```python
from build123d import *

# Parameters (mm, degrees)
BOSS_EXTRUDE1_DEPTH = 30
BOSS_EXTRUDE3_DEPTH = 5
BOSS_EXTRUDE4_DEPTH = 60
BOSS_EXTRUDE5_DEPTH = 5
RIB2_REACH          = 93.092
SKETCH12_WALL_W     = 244.715003534
SKETCH12_WALL_H     = 1.5
RIB4_REACH          = 88.249
SKETCH15_WALL_W     = 235.02855303
SKETCH15_WALL_H     = 1.5
FILLET2_R           = 6
FILLET3_R           = 3
FILLET4_R           = 5
FILLET6_R           = 1
CUT_EXTRUDE4_DEPTH  = 88.321245983
SKETCH17_R          = 12.5
CUT_EXTRUDE5_DEPTH  = 5
FILLET7_R           = 1
FILLET8_R           = 1


with BuildPart() as part:
    # Sketch1 → Boss-Extrude1 (new body)
    with BuildSketch(Plane.XY):
        Polygon((0, 0), (0, 50), (-12.5, 50), (-12.5, 25.213498553), (-10.5, 25.213498553), (-10.5, 48), (-6.7, 48), (-4, 43.5), (-4, 0), align=None)
    extrude(amount=BOSS_EXTRUDE1_DEPTH)

    # Sketch2 → Boss-Extrude3 (add)
    with BuildSketch(Plane(origin=(0, 0, 0), x_dir=(0, 0, -1), z_dir=(1, 0, 0))):
        with BuildLine():
            Line((-30, 20), (-30, 29.013878189))
            ThreePointArc((-30, 29.013878189), (-15, 37.5), (0, 29.013878189))
            Line((0, 29.013878189), (0, 20))
            Line((0, 20), (0, 10.986121811))
            ThreePointArc((0, 10.986121811), (-15, 2.5), (-30, 10.986121811))
            Line((-30, 10.986121811), (-30, 20))
        make_face()
    extrude(amount=BOSS_EXTRUDE3_DEPTH)

    # Sketch8 → Boss-Extrude4 (add)
    with BuildSketch(Plane(origin=(5, 0, 0), x_dir=(0, 0, -1), z_dir=(1, 0, 0))):
        with BuildLine():
            Line((-15.593853911, 21.273523821), (-14.406146089, 21.273523821))
            Line((-14.406146089, 21.273523821), (-8.660726074, 33.594616806))
            ThreePointArc((-8.660726074, 33.594616806), (-1.141807012, 25.740251485), (-0.904610688, 14.86969785))
            Line((-0.904610688, 14.86969785), (-10.032290508, 18.191901612))
            Line((-10.032290508, 18.191901612), (-19.967709492, 18.191901612))
            Line((-19.967709492, 18.191901612), (-29.095389312, 14.86969785))
            ThreePointArc((-29.095389312, 14.86969785), (-28.858192988, 25.740251485), (-21.339273926, 33.594616806))
            Line((-21.339273926, 33.594616806), (-15.593853911, 21.273523821))
        make_face()
    extrude(amount=BOSS_EXTRUDE4_DEPTH)

    # Sketch9 → Boss-Extrude5 (add)
    with BuildSketch(Plane(origin=(65, 0, 0), x_dir=(0, 0, -1), z_dir=(1, 0, 0))):
        with BuildLine():
            Line((-21.339273926, 33.594616806), (-22.39581958, 35.860386273))
            ThreePointArc((-22.39581958, 35.860386273), (-26.709477013, 33.005312303), (-30, 29.013878189))
            Line((-30, 29.013878189), (-27.857142857, 27.726181305))
            ThreePointArc((-27.857142857, 27.726181305), (-29.930908857, 21.438040583), (-29.095389312, 14.86969785))
            Line((-29.095389312, 14.86969785), (-19.967709492, 18.191901612))
            Line((-19.967709492, 18.191901612), (-10.032290508, 18.191901612))
            Line((-10.032290508, 18.191901612), (-0.904610688, 14.86969785))
            ThreePointArc((-0.904610688, 14.86969785), (-0.069091143, 21.438040583), (-2.142857143, 27.726181305))
            Line((-2.142857143, 27.726181305), (0, 29.013878189))
            ThreePointArc((0, 29.013878189), (-3.290522987, 33.005312303), (-7.60418042, 35.860386273))
            Line((-7.60418042, 35.860386273), (-8.660726074, 33.594616806))
            Line((-8.660726074, 33.594616806), (-14.406146089, 21.273523821))
            Line((-14.406146089, 21.273523821), (-15.593853911, 21.273523821))
            Line((-15.593853911, 21.273523821), (-21.339273926, 33.594616806))
        make_face()
    extrude(amount=BOSS_EXTRUDE5_DEPTH)

    # Sketch12 wall → Rib2 (add, up to next)
    with BuildSketch(Plane(origin=(35, 12.772029248, 23.163468829), x_dir=(0.991227900683, 0.1241932725, 0.045202654495), z_dir=(-0.132163720089, 0.931449543789, 0.33901990866)), mode=Mode.PRIVATE) as rib2_sk1:
        Rectangle(SKETCH12_WALL_W, SKETCH12_WALL_H)
    rib2_tool1 = extrude(rib2_sk1.sketch, amount=RIB2_REACH, mode=Mode.PRIVATE) - part.part
    add(rib2_tool1.solids().sort_by_distance((35, 12.772029248, 23.163468829))[0])

    # Sketch15 wall → Rib4 (add, up to next)
    with BuildSketch(Plane(origin=(35, 12.772029248, 6.836531171), x_dir=(0.991227900683, 0.1241932725, -0.045202654495), z_dir=(-0.132163720089, 0.931449543789, -0.33901990866)), mode=Mode.PRIVATE) as rib4_sk1:
        Rectangle(SKETCH15_WALL_W, SKETCH15_WALL_H)
    rib4_tool1 = extrude(rib4_sk1.sketch, amount=RIB4_REACH, mode=Mode.PRIVATE) - part.part
    add(rib4_tool1.solids().sort_by_distance((35, 12.772029248, 6.836531171))[0])

    # Fillet2
    fillet2_edges = [part.edges().sort_by_distance(p)[0] for p in [
        (0, 50, 15),
    ]]
    fillet(fillet2_edges, radius=FILLET2_R)

    # Fillet3
    fillet3_edges = [part.edges().sort_by_distance(p)[0] for p in [
        (-12.5, 50, 15),
    ]]
    fillet(fillet3_edges, radius=FILLET3_R)

    # Fillet4
    fillet4_edges = [part.edges().sort_by_distance(p)[0] for p in [
        (-2, 0, 0),
        (-2, 0, 30),
    ]]
    fillet(fillet4_edges, radius=FILLET4_R)

    # Fillet6
    # the kernel refuses this fillet: 1 mm, written as the material it adds along each edge
    with BuildSketch(Plane(origin=(67.5, 16.274284624, 25.236318868), x_dir=(-8.283054797608712e-12, -0.34202014332566627, 0.9396926207859093), z_dir=(-1.0, 2.8329715890524774e-12, -7.783525470878232e-12))) as fillet6_piece_1_section:
        with BuildLine():
            CenterArc((FILLET6_R, -FILLET6_R), FILLET6_R, 90, 90)
            Line((0, -FILLET6_R), (0, 0))
            Line((0, 0), (FILLET6_R, 0))
        make_face()
    fillet6_piece_1 = extrude(amount=65, mode=Mode.PRIVATE)
    fillet6_piece_1 = split(fillet6_piece_1, bisect_by=Plane(origin=(34.683018445, 12.397159057, 24.069843938), z_dir=(-0.13216372008897792, 0.9314495437888441, 0.33901990865994336)), keep=Keep.TOP, mode=Mode.PRIVATE)
    add(fillet6_piece_1)
    with BuildSketch(Plane(origin=(2.5, 16.787314839, 23.826779936), x_dir=(8.283054797608713e-12, 0.3420201433256657, -0.9396926207859096), z_dir=(1.0, -2.8329715890524774e-12, 7.783525470878232e-12))) as fillet6_piece_2_section:
        with BuildLine():
            CenterArc((FILLET6_R, -FILLET6_R), FILLET6_R, 90, 90)
            Line((0, -FILLET6_R), (0, 0))
            Line((0, 0), (FILLET6_R, 0))
        make_face()
    fillet6_piece_2 = extrude(amount=65, mode=Mode.PRIVATE)
    fillet6_piece_2 = split(fillet6_piece_2, bisect_by=Plane(origin=(4.790210247, 9.320920511, 20.868309995), z_dir=(-0.13216372008897792, 0.9314495437888441, 0.33901990865994336)), keep=Keep.TOP, mode=Mode.PRIVATE)
    add(fillet6_piece_2)
    with BuildSketch(Plane(origin=(67.5, 16.787314839, 6.173220063), x_dir=(8.283047858714808e-12, 0.3420201433256657, 0.9396926207859096), z_dir=(-1.0, 2.8329692158109876e-12, 7.783518950450833e-12))) as fillet6_piece_3_section:
        with BuildLine():
            CenterArc((FILLET6_R, -FILLET6_R), FILLET6_R, 90, 90)
            Line((0, -FILLET6_R), (0, 0))
            Line((0, 0), (FILLET6_R, 0))
        make_face()
    fillet6_piece_3 = extrude(amount=65, mode=Mode.PRIVATE)
    fillet6_piece_3 = split(fillet6_piece_3, bisect_by=Plane(origin=(34.683018444, 13.067468711, 7.7718167), z_dir=(-0.13216372008897792, 0.9314495437888441, -0.33901990865994336)), keep=Keep.TOP, mode=Mode.PRIVATE)
    add(fillet6_piece_3)
    with BuildSketch(Plane(origin=(2.5, 16.274284624, 4.763681132), x_dir=(-8.283047858714808e-12, -0.342020143325666, -0.9396926207859094), z_dir=(1.0, -2.8329692158109876e-12, -7.783518950450833e-12))) as fillet6_piece_4_section:
        with BuildLine():
            CenterArc((FILLET6_R, -FILLET6_R), FILLET6_R, 90, 90)
            Line((0, -FILLET6_R), (0, 0))
            Line((0, 0), (FILLET6_R, 0))
        make_face()
    fillet6_piece_4 = extrude(amount=65, mode=Mode.PRIVATE)
    fillet6_piece_4 = split(fillet6_piece_4, bisect_by=Plane(origin=(4.790210247, 8.653026917, 7.296667437), z_dir=(-0.13216372008897792, 0.9314495437888441, -0.33901990865994336)), keep=Keep.TOP, mode=Mode.PRIVATE)
    add(fillet6_piece_4)

    # Sketch16 → Cut-Extrude4 (cut, through all)
    with BuildSketch(Plane(origin=(5, 0, 0), x_dir=(0, 0, -1), z_dir=(1, 0, 0))):
        Polygon((-19.967709492, 16.824178281), (-10.106442475, 16.824178281), (-8.435471613, 16.167725442), (-12.864533528, 4.893749658), (-16.690177608, 4.893749658), (-21.504850857, 16.167725442), align=None)
    extrude(amount=-CUT_EXTRUDE4_DEPTH, mode=Mode.SUBTRACT)

    # Sketch17 → Cut-Extrude5 (cut)
    with BuildSketch(Plane.ZY.offset(4)):
        with Locations((15, 20)):
            Circle(SKETCH17_R)
    extrude(amount=-CUT_EXTRUDE5_DEPTH, mode=Mode.SUBTRACT)

    # Fillet7
    fillet7_edges = [part.edges().sort_by_distance(p)[0] for p in [
        (-12.5, 25.213498553, 15),
    ]]
    fillet(fillet7_edges, radius=FILLET7_R)

    # Fillet8
    fillet8_edges = [part.edges().sort_by_distance(p)[0] for p in [
        (0, 37.5, 15),
        (0, 2.5, 15),
    ]]
    fillet(fillet8_edges, radius=FILLET8_R)


solid = part.part
```
The model under review builds one solid part; all positions refer to its coordinate system, in mm. A direction names the side the tool comes from. Give positions to 0.01 mm unless a question says otherwise; leave off trailing zeros. Write each loop counter-clockwise with the first axis right and the second up, starting at its lowest first coordinate (ties: lowest second). Pieces come first, ordered by that corner, then holes. Notation, with made-up numbers: (81, 38) -> (115, 38) arc R29 cw to (115, 76) -> close; hole circle Ø9 at (73, 64.25). An arc over 180 degrees is marked (long way). Put each result on its own line as item: value.
(1) The part is to be moulded in two halves that separate along X. For faces 4 (the flat face through (5, 30, 15)), 5 (the cylindrical face through (-11.6, 49.14, 15.21)), 6 (the flat face through (37, 18.192, 15)), 7 (the flat face through (0, 40, 15)), say which applies: pulls with the +X half, pulls with the -X half, needs draft (parallel to the pull), parting line crosses it, or undercut.
Results are:
face 4: undercut
face 5: pulls with the -X half
face 6: needs draft
face 7: pulls with the +X half
(2) Tool access review of faces 1 (the flat face through (3.03, 16.5, 9.28)), 2 (the cylindrical face through (2.97, 37.5, 15.25)), 3 (the flat face through (-4, 32, 8)): name each direction out of +Z, -Z, +X, -X, +Y, -Y from which nothing blocks a thin tool from reaching the whole face with its end or side.
Results are:
face 1: +X, -X
face 2: +X, +Y
face 3: +Z, -Z, -Y
(3) To check wall thickness, follow probe 1 along X at (y, z) = (33, 5); probe 2 along Z at (x, y) = (-1, 20); probe 3 along X at (y, z) = (43.5, 26). State the ranges of each line that lie inside material, in increasing order. Write a range as from..to.
Results are:
probe 1: -12.5..-10.5, -4..5, 65..70
probe 2: 0..2.5, 27.5..30
probe 3: -12.5..-10.5, -4..0
(4) We need section A-A, the plane y = 12.5. Give the boundary of the cut face in (x, z), and give its area (3 significant figures).
Results are:
outline: (-4, 0) -> (5, 0) -> (5, 6.14) -> (34.88, 6.14) -> (30.78, 7.73) -> (5, 7.73) -> (5, 9.88) -> (1, 9.88) -> (1, 5) -> (-4, 5) -> close; (-4, 25) -> (1, 25) -> (1, 19.94) -> (5, 19.94) -> (5, 22.27) -> (30.78, 22.27) -> (34.88, 23.86) -> (5, 23.86) -> (5, 30) -> (-4, 30) -> close
area: 219 mm²
(5) We need section B-B, the plane x = 36.5. Give the boundary of the cut face in (y, z).
Results are:
outline: (12.7, 6.06) -> (15.33, 5.11) arc R1 cw to (15.93, 3.82) -> (14.87, 0.9) arc R15 ccw to (33.59, 8.66) -> (21.27, 14.41) -> (21.27, 15.59) -> (33.59, 21.34) arc R15 ccw to (14.87, 29.1) -> (15.93, 26.18) arc R1 cw to (15.33, 24.89) -> (12.7, 23.94) -> (13.22, 22.53) -> (15.85, 23.48) arc R1 cw to (17.13, 22.89) -> (18.19, 19.97) -> (18.19, 10.03) -> (17.13, 7.11) arc R1 cw to (15.85, 6.52) -> (13.22, 7.47) -> close
(6) We need section C-C, the plane x = 61. Give the boundary of the cut face in (y, z), and give its area (3 significant figures).
Results are:
outline: (14.87, 0.9) arc R15 ccw to (33.59, 8.66) -> (21.27, 14.41) -> (21.27, 15.59) -> (33.59, 21.34) arc R15 ccw to (14.87, 29.1) -> (15.93, 26.18) arc R1 cw to (15.73, 25.16) -> (16.33, 23.54) arc R1 cw to (17.13, 22.89) -> (18.19, 19.97) -> (18.19, 10.03) -> (17.13, 7.11) arc R1 cw to (16.33, 6.46) -> (15.73, 4.84) arc R1 cw to (15.93, 3.82) -> close
area: 346 mm²
(7) For pin 1 Ø1.1 at (x, z) = (0, 15) entering from +Y; pin 2 Ø3 at (y, z) = (3, 20) entering from +X; pin 3 Ø5 at (x, z) = (4.5, 8.5) entering from -Y, all flat-tipped, find the tip position at first contact; note any pin that passes through.
Results are:
pin 1: y = 46.51
pin 2: x = 5
pin 3: y = 2.96
